from build123d import *

# Parameters (mm, degrees)
SKETCH1_W           = 50.8
SKETCH1_H           = 25.4
BOSS_EXTRUDE1_DEPTH = 44.45
SHELL1_T            = -1.5875
SKETCH2_R           = 2.4892
CUT_EXTRUDE1_DEPTH  = 26.4
SKETCH3_R           = 2.4892
CUT_EXTRUDE2_DEPTH  = 51.8


with BuildPart() as part:
    # Sketch1 → Boss-Extrude1 (new body, symmetric)
    with BuildSketch(Plane(origin=(0, 0, 0), x_dir=(0, 0, -1), z_dir=(1, 0, 0))):
        with Locations((25.4, 12.7)):
            Rectangle(SKETCH1_W, SKETCH1_H)
    extrude(amount=BOSS_EXTRUDE1_DEPTH, both=True)

    # Shell1
    shell1_openings = [part.faces().sort_by_distance(p)[0] for p in [
        (44.45, 12.7, -25.4),
        (-44.45, 12.7, -25.4),
    ]]
    offset(amount=SHELL1_T, openings=shell1_openings, kind=Kind.INTERSECTION)

    # Sketch2 → Cut-Extrude1 (cut, through all)
    with BuildSketch(Plane(origin=(0, 25.4, 0), x_dir=(1, 0, 0), z_dir=(0, 1, 0))):
        with Locations((-31.75, 25.4)):
            Circle(SKETCH2_R)
        with Locations((-31.75, 12.7)):
            Circle(SKETCH2_R)
        with Locations((-31.75, 38.1)):
            Circle(SKETCH2_R)
    cut_extrude1 = extrude(amount=-CUT_EXTRUDE1_DEPTH, mode=Mode.SUBTRACT)

    # Sketch3 → Cut-Extrude2 (cut, through all)
    with BuildSketch(Plane.XY):
        with Locations((-31.75, 12.7)):
            Circle(SKETCH3_R)
    cut_extrude2 = extrude(amount=-CUT_EXTRUDE2_DEPTH, mode=Mode.SUBTRACT)

    # Mirror1: Cut-Extrude1, Cut-Extrude2 across plane
    add(cut_extrude1.mirror(Plane(origin=(0, 0, 0), x_dir=(0, 0, 1), z_dir=(1, 0, 0))), mode=Mode.SUBTRACT)
    add(cut_extrude2.mirror(Plane(origin=(0, 0, 0), x_dir=(0, 0, 1), z_dir=(1, 0, 0))), mode=Mode.SUBTRACT)


solid = part.part
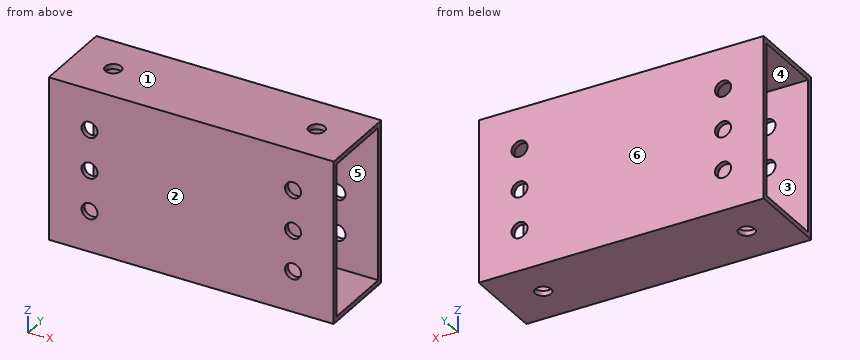
The listing builds one solid part. Answer for the finished solid, in the listing's coordinates (mm). Face numbers are marked on the shaded views. A direction names the side the tool comes from. Coordinates: 2 decimals unless noted, no trailing zeros. Write each loop counter-clockwise with the first axis right and the second up, starting at its lowest first coordinate (ties: lowest second). Pieces come first, ordered by that corner, then holes. Notation, with made-up numbers: M -2,68 L 54,68 A19 ccw 54,102 Z; hole C 36,78.25 d2. An arc over 180 degrees is marked long. Put each result on its own line as item: value. Start each with the question number.
1. A cutting plane is placed at C-C on z = -7.5. Write down the section's boundary in (x, y).
2. A cutting plane is placed at A-A on y = 4. Write down the section's boundary in (x, z).
3. A cutting plane is placed at D-D on z = -38.1. Write down the section's boundary in (x, y), then the cut area to 3 significant figures.
4. Consider line 1 (Z direction, x = -31.75, y = 1); line 2 (X direction, y = 24.2, z = -25.4); line 3 (Y direction, x = 20.5, z = -18.5). Determine where each line is inside the solid, lowest interval first. Write a range as from..to.
5. For a pull along Y with two mould halves and no side action, classify the marked faces 1, 2, 3 and 4 as pulls with the +Y half, pulls with the -Y half, needs draft (parallel to the pull), parting line crosses it, or undercut.
6. Which of the six approach directions +Z, -Z, +X, -X, +Y, -Y give full straight-line access (tool end or side, diameter ignored) to the marked faces 5 and 6?
7. A cutting plane is placed at B-B on x = 3.5. Write down the section's boundary in (y, z).
8. A flat-ended cylindrical pin translates along its axis: P1, Ø4, axis at x = -31.75, z = -38.1, coming from the +Y side. Find the tip coordinate at first contact, or state that the pin passes through.
Resolved:
1. outline: M -44.45,0 L 44.45,0 L 44.45,1.59 L -44.45,1.59 Z; M -44.45,23.81 L 44.45,23.81 L 44.45,25.4 L -44.45,25.4 Z
2. outline: M -44.45,-50.8 L 44.45,-50.8 L 44.45,-49.21 L -44.45,-49.21 Z; M -44.45,-1.59 L 44.45,-1.59 L 44.45,0 L -44.45,0 Z
3. outline: M -44.45,0 L -34.24,0 L -34.24,1.59 L -44.45,1.59 Z; M -44.45,23.81 L -34.24,23.81 L -34.24,25.4 L -44.45,25.4 Z; M -29.26,0 L 29.26,0 L 29.26,1.59 L -29.26,1.59 Z; M -29.26,23.81 L 29.26,23.81 L 29.26,25.4 L -29.26,25.4 Z; M 34.24,0 L 44.45,0 L 44.45,1.59 L 34.24,1.59 Z; M 34.24,23.81 L 44.45,23.81 L 44.45,25.4 L 34.24,25.4 Z
3. area: 251 mm2
4. line 1: z = -50.8..-40.59, -35.61..-27.89, -22.91..-15.19, -10.21..0
4. line 2: x = -44.45..-34.24, -29.26..29.26, 34.24..44.45
4. line 3: y = 0..1.59, 23.81..25.4
5. face 1: needs draft
5. face 2: pulls with the -Y half
5. face 3: undercut
5. face 4: undercut
6. face 5: +X, -X
6. face 6: +Z, -Z, +X, -X, +Y
7. outline: M 0,-50.8 L 25.4,-50.8 L 25.4,0 L 0,0 Z; hole M 1.59,-49.21 L 23.81,-49.21 L 23.81,-1.59 L 1.59,-1.59 Z
8. P1: passes through
